Geometry: see drawing. Coordinates: mm, zero at the bounding-box minimum. A direction names the side the tool comes from. Round coordinates to 2 decimals unless told otherwise and drop trailing zeros. Order: outer loops, then holes, each group sorted by start corner. A loop starts at its lowest first (then second) coordinate and runs counter-clockwise, first axis right, second up. Notation, with made-up numbers: M 31.5,47.25 L 47.5,47.25 A21 ccw 47.5,67.25 Z; hole C -28,-34 d9. An arc over 180 degrees is marked long. Answer in a Markdown table with one row per item. Add a question column.
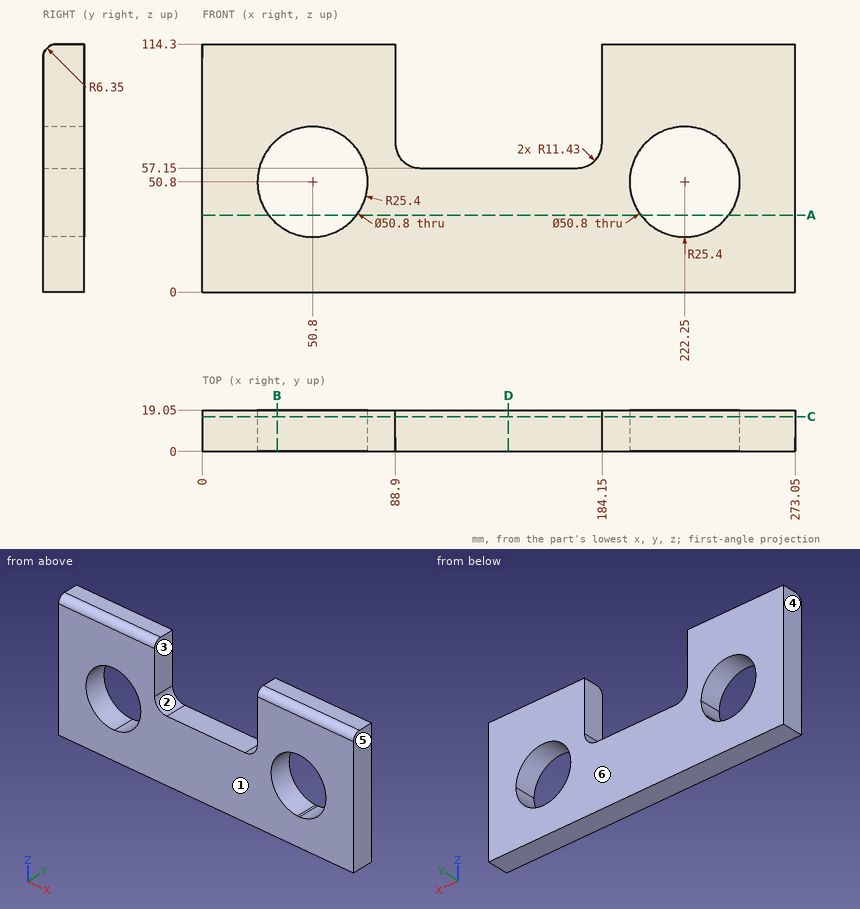
(1) Cut plane B-B (x = 34.5). Return loops of the section in (y, z), and give its area (3 significant figures).
(2) Cut plane C-C (y = 16). Return loops of the section in (x, z), and give its area (3 significant figures).
(3) Draft query along X for the marked faces 3, 4, 5 and 6. Return one class per face: +X half, -X half, draft (parallel to the pull), parting line (faces both ways), or undercut.
(4) Pin query (flat end, axial travel): pin 1 (9.5 mm diameter, centred on x = 127.5, y = 12.5, fed in from +Z). Return the tip coordinate at first contact, or that it passes through.
(5) Line query: line 1 (X direction, y = 14.25, z = 50.8); line 2 (X direction, y = 8.75, z = 108.5); line 3 (Z direction, x = 50.8, y = 6.5). Output: solid intervals per line, ascending. Write a range as from..to.
(6) Cut plane A-A (z = 35.5). Return loops of the section in (x, y).
(7) Cut plane D-D (x = 141). Return loops of the section in (y, z), and give its area (3 significant figures).
(8) Access query for the marked faces 1 and 2. Directions: +Z, -Z, +X, -X, +Y, -Y. A direction counts if a zero-diameter tool reaches every point of the face in a straight line with its end or side. Return the directions, or none.
Answer list:
| question | item | result |
|---|---|---|
| 1 | outline | M 0,0 L 19.05,0 L 19.05,31.32 L 0,31.32 Z; M 0,70.28 L 19.05,70.28 L 19.05,114.3 L 6.35,114.3 A6.35 ccw 0,107.95 Z |
| 1 | area | 1,430 mm² |
| 2 | outline | M 0,0 L 273.05,0 L 273.05,114.3 L 184.15,114.3 L 184.15,68.58 A11.43 cw 172.72,57.15 L 100.33,57.15 A11.43 cw 88.9,68.58 L 88.9,114.3 L 0,114.3 Z; hole C 50.8,50.8 d50.8; hole C 222.25,50.8 d50.8 |
| 2 | area | 21,800 mm² |
| 3 | face 3 | undercut |
| 3 | face 4 | -X half |
| 3 | face 5 | +X half |
| 3 | face 6 | draft |
| 4 | pin 1 | z = 57.15 |
| 5 | line 1 | 0..25.4, 76.2..196.85, 247.65..273.05 |
| 5 | line 2 | 0..88.9, 184.15..273.05 |
| 5 | line 3 | 0..25.4, 76.2..114.3 |
| 6 | outline | M 0,0 L 30.53,0 L 30.53,19.05 L 0,19.05 Z; M 71.07,0 L 201.98,0 L 201.98,19.05 L 71.07,19.05 Z; M 242.52,0 L 273.05,0 L 273.05,19.05 L 242.52,19.05 Z |
| 7 | outline | M 0,0 L 19.05,0 L 19.05,57.15 L 0,57.15 Z |
| 7 | area | 1,090 mm² |
| 8 | face 1 | +Z, -Z, +X, -X, -Y |
| 8 | face 2 | +Z, +Y, -Y |
